Input: dimensioned drawing with shaded views. Units: mm. Origin: part minimum x, y, z. A direction names the side the tool comes from. Round coordinates to 2 decimals unless told otherwise and drop trailing zeros. Loops run counter-clockwise (first coordinate to the right, second up) from the corner with the lowest first, then second, coordinate; pieces in that order, holes last. Notation, with made-up numbers: M -4,79 L 33,79 A19 ccw 33,93 Z; hole C 81,-18.5 d4. An arc over 180 degrees is marked long. Return JSON: item names as keys, results as strings.
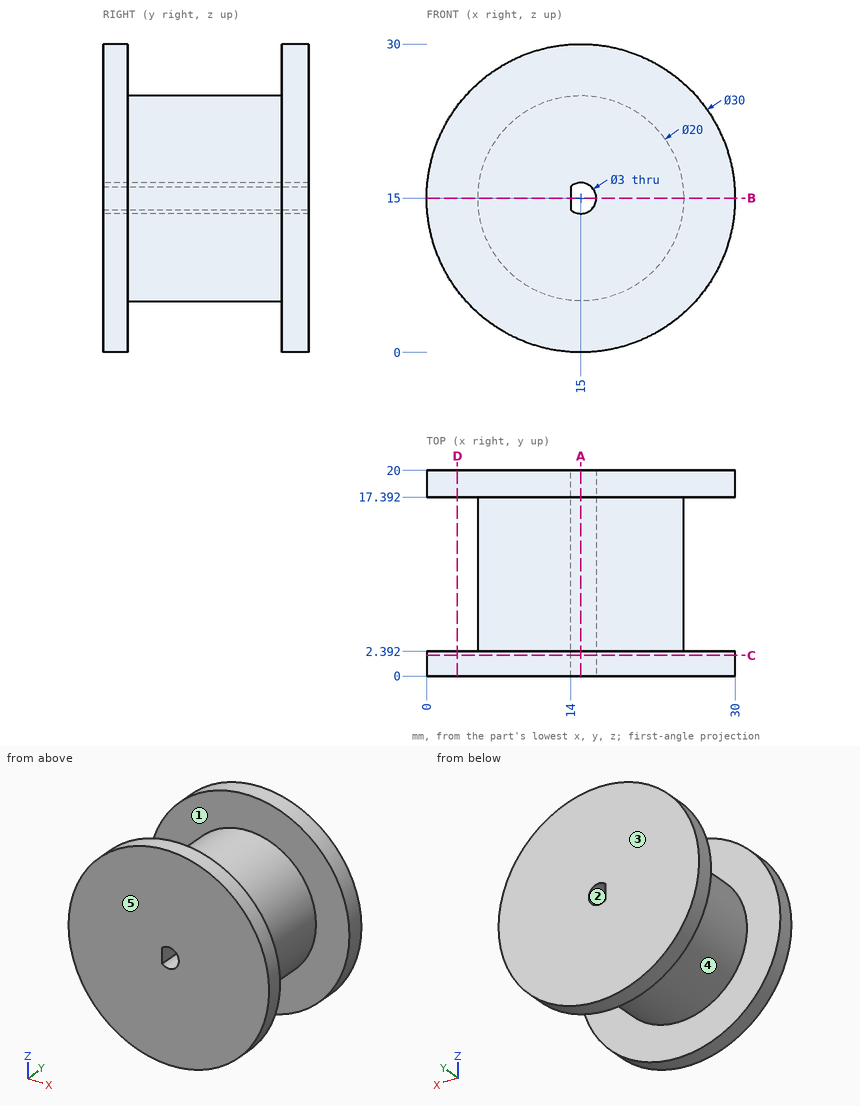
Q1. Section query B-B (z = 15). Output: boundary loops of the cut face in (x, y).
Determined:
{"outline": "M 0,0 L 14,0 L 14,20 L 0,20 L 0,17.39 L 5,17.39 L 5,2.39 L 0,2.39 Z; M 16.5,0 L 30,0 L 30,2.39 L 25,2.39 L 25,17.39 L 30,17.39 L 30,20 L 16.5,20 Z"}
Q2. Reachability of the marked faces 4 and 5 from +Z, -Z, +X, -X, +Y, -Y: full face, straight path, thin tool, end or side. Return the list, or none.
Determined:
{"face 4": "none", "face 5": "+Z, -Z, +X, -X, -Y"}
Q3. Pull-direction query (Y, two-part tool) for the marked faces 1, 2 and 3; classes: pulls with the +Y half, pulls with the -Y half, needs draft (parallel to the pull), parting line crosses it, or undercut.
Determined:
{"face 1": "undercut", "face 2": "needs draft", "face 3": "pulls with the +Y half"}
Q4. Section query C-C (y = 2). Output: boundary loops of the cut face in (x, z).
Determined:
{"outline": "C 15,15 d30; hole M 14,13.88 A1.5 ccw long 14,16.12 Z"}
Q5. Section query A-A (x = 15). Output: boundary loops of the cut face in (y, z).
Determined:
{"outline": "M 0,0 L 2.39,0 L 2.39,5 L 17.39,5 L 17.39,0 L 20,0 L 20,13.5 L 0,13.5 Z; M 0,16.5 L 20,16.5 L 20,30 L 17.39,30 L 17.39,25 L 2.39,25 L 2.39,30 L 0,30 Z"}
Q6. Material intervals for L1, parallel to Y at x = 28.5, z = 17; L2, parallel to X at y = 7, z = 15; L3, parallel to Z at x = 15, y = 15.25, sorted ascending.
Determined:
{"L1": "y = 0 to 2.39, 17.39 to 20", "L2": "x = 5 to 14, 16.5 to 25", "L3": "z = 5 to 13.5, 16.5 to 25"}
Q7. Section query D-D (x = 3). Output: boundary loops of the cut face in (y, z).
Determined:
{"outline": "M 0,6 L 2.39,6 L 2.39,24 L 0,24 Z; M 17.39,6 L 20,6 L 20,24 L 17.39,24 Z"}
Q8. Pin query (flat end, axial travel): pin 1 (2 mm diameter, centred on y = 13.5, z = 15.5, fed in from +X); pin 2 (1 mm diameter, centred on x = 6, y = 8.5, fed in from -Z); pin 3 (6 mm diameter, centred on x = 5.5, y = 11, fed in from -Z). Return the tip coordinate at first contact, or that it passes through.
Determined:
{"pin 1": "stops at x = 25", "pin 2": "stops at z = 9.73", "pin 3": "stops at z = 7.4"}
